Part model, mm, in its own coordinate system. A direction names the side the tool comes from. Round coordinates to 2 decimals unless told otherwise and drop trailing zeros. Loops run counter-clockwise (first coordinate to the right, second up) from the corner with the lowest first, then second, coordinate; pieces in that order, holes last. Notation, with made-up numbers: (-16.5, 81.25) -> (12.5, 81.25) arc R20 cw to (12.5, 105.25) -> close; hole circle Ø11 at (67.25, -39). An arc over 180 degrees is marked (long way). Answer as a JSON object with one key per item and string values. Group by question number.
from build123d import *

# Parameters (mm, degrees)
BOSS_EXTRUDE1_DEPTH = 17
CHAMFER1_SIZE       = 0.5
CUT_EXTRUDE1_DEPTH  = 13
BOSS_EXTRUDE2_START = -2
BOSS_EXTRUDE2_DEPTH = 2
SKETCH2_R           = 1.5499999999999992
SKETCH2_R_2         = 1.550000000000003
SKETCH2_R_3         = 2.5
CUT_EXTRUDE2_DEPTH  = 2
BOSS_EXTRUDE3_DEPTH = 5
FILLET1_R           = 2
FILLET2_R           = 0.5
CHAMFER3_SIZE       = 0.5
CHAMFER3_SIZE2      = 3
CHAMFER4_SIZE       = 1


with BuildPart() as part:
    # Sketch1 → Boss-Extrude1 (new body)
    with BuildSketch(Plane(origin=(0, 0, 0), x_dir=(1, 0, 0), z_dir=(0, 1, 0))):
        with BuildLine():
            ThreePointArc((13.418634843133532, 19.2879126019326), (5.33e-15, 27.035165040773038), (-13.418634843133521, 19.287912601932604))
            Line((-13.418634843133521, 19.2879126019326), (-23.413139720814414, 1.9769223572943453))
            ThreePointArc((-23.413139720814414, 1.976922357294347), (-23.413139720814407, -13.517582520386524), (-9.994504877680875, -21.264834959226956))
            Line((-9.994504877680875, -21.264834959226956), (9.994504877680878, -21.26483495922696))
            ThreePointArc((9.994504877680878, -21.26483495922696), (23.413139720814414, -13.517582520386526), (23.41313972081442, 1.9769223572943506))
            Line((23.41313972081442, 1.9769223572943488), (13.418634843133532, 19.2879126019326))
        make_face()
        with BuildLine():
            Line((-11.469734859267339, 10.663506392859015), (-11.902747561159552, 10.91350639285901))
            Line((-11.902747561159554, 10.91350639285901), (-10.975952641916443, 12.518762281184774))
            Line((-10.975952641916448, 12.518762281184776), (-12.361593287971548, 13.318762281184778))
            Line((-12.361593287971548, 13.318762281184778), (-11.561593287971546, 14.70440292723988))
            Line((-11.561593287971546, 14.70440292723988), (-10.17595264191644, 13.904402927239877))
            Line((-10.175952641916442, 13.904402927239877), (-8.655495122319113, 16.537912601932604))
            ThreePointArc((-8.655495122319113, 16.537912601932604), (1.33e-15, 21.535165040773038), (8.655495122319117, 16.537912601932604))
            Line((8.655495122319117, 16.537912601932604), (10.175952641916444, 13.904402927239877))
            Line((10.175952641916444, 13.904402927239877), (11.561593287971549, 14.70440292723988))
            Line((11.561593287971549, 14.70440292723988), (12.361593287971552, 13.318762281184778))
            Line((12.361593287971552, 13.318762281184778), (10.975952641916452, 12.518762281184776))
            Line((10.975952641916447, 12.518762281184772), (11.902747561159558, 10.91350639285901))
            Line((11.902747561159556, 10.913506392859007), (11.46973485926734, 10.663506392859015))
            Line((11.46973485926734, 10.663506392859015), (14.969734859267339, 4.601328566367944))
            Line((14.969734859267339, 4.601328566367944), (15.402747561159552, 4.851328566367944))
            Line((15.402747561159552, 4.8513285663679415), (18.64999999999999, -0.7730776427056512))
            ThreePointArc((18.64999999999999, -0.7730776427056494), (18.65, -10.767582520386522), (9.994504877680878, -15.764834959226958))
            Line((9.994504877680878, -15.76483495922696), (-9.994504877680871, -15.76483495922696))
            ThreePointArc((-9.994504877680868, -15.76483495922696), (-18.64999999999999, -10.767582520386524), (-18.64999999999999, -0.7730776427056494))
            Line((-18.64999999999999, -0.7730776427056512), (-15.402747561159547, 4.851328566367947))
            Line((-15.40274756115955, 4.851328566367947), (-14.969734859267337, 4.601328566367946))
            Line((-14.969734859267337, 4.601328566367946), (-11.469734859267339, 10.663506392859015))
        make_face(mode=Mode.SUBTRACT)
        with BuildLine():
            Line((13.63479836872844, 11.913506392859018), (14.609798368728441, 10.224756855479358))
            ThreePointArc((14.609798368728436, 10.224756855479354), (16.727137744594316, 9.657417479613473), (16.159798368728428, 7.540078103747593))
            Line((16.15979836872844, 7.5400781037476), (17.13479836872844, 5.851328566367942))
            Line((17.13479836872844, 5.851328566367942), (16.268772964944, 5.351328566367942))
            Line((16.268772964944, 5.351328566367942), (12.768772964944, 11.413506392859018))
            Line((12.768772964944, 11.413506392859018), (13.63479836872844, 11.913506392859018))
        make_face(mode=Mode.SUBTRACT)
        with BuildLine():
            Line((-13.634798368728436, 11.913506392859018), (-12.768772964943997, 11.413506392859018))
            Line((-12.768772964943997, 11.413506392859018), (-16.268772964944, 5.351328566367942))
            Line((-16.268772964944, 5.351328566367942), (-17.13479836872844, 5.851328566367942))
            Line((-17.13479836872844, 5.851328566367942), (-16.159798368728442, 7.540078103747597))
            ThreePointArc((-16.159798368728435, 7.540078103747593), (-16.727137744594312, 9.65741747961347), (-14.60979836872844, 10.224756855479354))
            Line((-14.609798368728441, 10.224756855479356), (-13.634798368728436, 11.913506392859018))
        make_face(mode=Mode.SUBTRACT)
    extrude(amount=BOSS_EXTRUDE1_DEPTH)

    # Chamfer1
    chamfer1_edges = [part.edges().sort_by_distance(p)[0] for p in [
        (-10.175952641916442, 8.5, -13.904402927239877),
        (-10.975952641916447, 8.5, -12.518762281184774),
        (10.97595264191645, 8.5, -12.518762281184774),
        (10.175952641916444, 8.5, -13.904402927239877),
    ]]
    chamfer(chamfer1_edges, length=CHAMFER1_SIZE)

    # Sketch1<3> → Cut-Extrude1 (cut)
    with BuildSketch(Plane(origin=(0, 0, 0), x_dir=(1, 0, 0), z_dir=(0, 1, 0))):
        Polygon((-12.585760263051778, 10.7304936909668), (-13.018772964943997, 10.9804936909668), (-13.518772964943999, 10.114468287182358), (-13.085760263051776, 9.86446828718236), align=None)
        Polygon((-15.08576026305178, 6.400366672044599), (-15.518772964944, 6.650366672044602), (-16.018772964944, 5.784341268260162), (-15.585760263051782, 5.53434126826016), align=None)
        Polygon((13.518772964944, 10.114468287182358), (13.018772964944, 10.9804936909668), (12.585760263051782, 10.7304936909668), (13.08576026305178, 9.86446828718236), align=None)
        Polygon((16.018772964944, 5.784341268260162), (15.518772964944, 6.6503666720445995), (15.085760263051784, 6.400366672044599), (15.585760263051785, 5.53434126826016), align=None)
    extrude(amount=CUT_EXTRUDE1_DEPTH, mode=Mode.SUBTRACT)

    # Sketch1<4> → Boss-Extrude2 (add)
    with BuildSketch(Plane(origin=(0, 0, 0), x_dir=(1, 0, 0), z_dir=(0, 1, 0)).offset(BOSS_EXTRUDE2_START)):
        with BuildLine():
            Line((-13.418634843133521, 19.2879126019326), (-23.413139720814414, 1.976922357294346))
            ThreePointArc((-23.413139720814414, 1.976922357294346), (-23.413139720814407, -13.517582520386522), (-9.994504877680875, -21.264834959226956))
            Line((-9.994504877680875, -21.264834959226956), (9.994504877680878, -21.26483495922696))
            ThreePointArc((9.994504877680878, -21.26483495922696), (23.413139720814414, -13.517582520386522), (23.41313972081442, 1.9769223572943484))
            Line((23.41313972081442, 1.9769223572943484), (13.418634843133532, 19.2879126019326))
            ThreePointArc((13.418634843133532, 19.2879126019326), (3.63e-15, 27.035165040773038), (-13.418634843133521, 19.2879126019326))
        make_face()
    extrude(amount=BOSS_EXTRUDE2_DEPTH)

    # Sketch2 → Cut-Extrude2 (cut)
    # profile 1 of 4: a face of its own
    with BuildSketch(Plane.XZ.offset(2)):
        with Locations(Location((-15.384798368728436, -8.882417479613482, 0), (0, 0, 270))):
            Circle(SKETCH2_R)
    # profile 2 of 4: a face of its own
    with BuildSketch(Plane.XZ.offset(2)):
        with Locations(Location((15.38479836872844, -8.882417479613482, 0), (0, 0, 270))):
            Circle(SKETCH2_R_2)
    # profile 3 of 4: a face of its own
    with BuildSketch(Plane.XZ.offset(2)):
        with Locations(Location((0, 0, 0), (0, 0, 270))):
            Circle(SKETCH2_R_3)
    # profile 4 of 4: a face of its own
    with BuildSketch(Plane.XZ.offset(2)):
        Polygon((5.499999999999999, 21.264834959226956), (5.5, 25.264834959226956), (-5.5, 25.264834959226956), (-5.499999999999999, 21.264834959226956), align=None)
        with BuildLine():
            Line((-1.4999999999999987, 24.264834959226945), (1.4999999999999987, 24.264834959226945))
            ThreePointArc((1.4999999999999987, 24.264834959226945), (2.7499999999999916, 23.014834959226953), (1.4999999999999987, 21.76483495922696))
            Line((1.4999999999999987, 21.76483495922696), (-1.4999999999999987, 21.76483495922696))
            ThreePointArc((-1.4999999999999987, 21.76483495922696), (-2.7499999999999916, 23.014834959226953), (-1.4999999999999987, 24.264834959226945))
        make_face(mode=Mode.SUBTRACT)
    extrude(amount=-CUT_EXTRUDE2_DEPTH, mode=Mode.SUBTRACT)

    # Sketch2<2> → Boss-Extrude3 (add)
    with BuildSketch(Plane.XZ.offset(2)):
        Polygon((-5.499999999999999, 21.264834959226956), (5.499999999999999, 21.264834959226956), (5.5, 25.264834959226956), (-5.5, 25.264834959226956), align=None)
        with BuildLine():
            ThreePointArc((-1.499999999999999, 21.76483495922696), (-2.7499999999999916, 23.014834959226953), (-1.4999999999999987, 24.264834959226945))
            Line((-1.4999999999999987, 24.264834959226945), (1.4999999999999987, 24.264834959226945))
            ThreePointArc((1.499999999999999, 24.264834959226945), (2.7499999999999916, 23.014834959226953), (1.4999999999999987, 21.76483495922696))
            Line((1.4999999999999987, 21.76483495922696), (-1.4999999999999987, 21.76483495922696))
        make_face(mode=Mode.SUBTRACT)
    extrude(amount=-BOSS_EXTRUDE3_DEPTH)

    # Fillet1
    fillet1_edges = [part.edges().sort_by_distance(p)[0] for p in [
        (5.499999999999999, 0.5, 21.264834959226956),
        (-5.499999999999999, 0.5, 21.264834959226956),
    ]]
    fillet(fillet1_edges, radius=FILLET1_R)
    fillet1_2_edges = [part.edges().sort_by_distance(p)[0] for p in [
        (5.5, 0.5, 25.264834959226956),
        (-5.5, 0.5, 25.264834959226956),
    ]]
    fillet(fillet1_2_edges, radius=FILLET1_R - 0.0001)  # a hair under: the kernel refuses the full size

    # Fillet2
    fillet2_edges = [part.edges().sort_by_distance(p)[0] for p in [
        (0, 3, 24.264834959226945),
        (2.7499999999999916, 3, 23.014834959226953),
        (-2.7499999999999916, 3, 23.014834959226953),
        (0, 3, 21.76483495922696),
    ]]
    fillet(fillet2_edges, radius=FILLET2_R - 0.0001)  # a hair under: the kernel refuses the full size

    # Chamfer3
    chamfer3_edges = [part.edges().sort_by_distance(p)[0] for p in [
        (13.21973485926734, 17, -7.63241747961348),
        (-13.219734859267337, 17, -7.63241747961348),
        (14.518772964943999, 17, -8.38241747961348),
        (-14.518772964943999, 17, -8.38241747961348),
    ]]
    chamfer3_side = [part.faces().sort_by_distance(p)[0] for p in [
        (-12.172522474712478, 17, -11.850756469441762),
    ]]
    chamfer(chamfer3_edges, length=CHAMFER3_SIZE, length2=CHAMFER3_SIZE2, reference=chamfer3_side[0])

    # Chamfer4
    chamfer4_edges = [part.edges().sort_by_distance(p)[0] for p in [
        (1.78e-15, 17, 21.26483495922696),
        (23.413139720814414, 17, 13.517582520386522),
        (18.415887281973976, 17, -10.632417479613474),
        (4.44e-15, 17, -27.035165040773038),
        (-18.415887281973966, 17, -10.632417479613473),
        (-23.413139720814407, 17, 13.517582520386526),
        (5.33e-15, -2, -27.035165040773038),
        (23.413139720814414, -2, 13.517582520386526),
        (-8.747252438840437, -2, 21.264834959226956),
        (-23.413139720814407, -2, 13.517582520386524),
        (-18.415887281973966, -2, -10.632417479613473),
        (18.415887281973976, -2, -10.632417479613474),
        (8.747252438840441, -2, 21.26483495922696),
        (0, -2, 25.264834959226956),
        (-4.9142428516949765, -2, 24.67907781092193),
        (4.914242851694976, -2, 24.67907781092193),
        (6.085786437626905, -2, 21.850621396853864),
        (-6.085786437626905, -2, 21.85062139685386),
    ]]
    chamfer(chamfer4_edges, length=CHAMFER4_SIZE - 0.0001)  # a hair under: the kernel refuses the full size


solid = part.part
Item 1: Band-saw the part on A-A, the plane x = 0. Count the separate pieces of the cut face and the enclosed holes in it, plus the area to 3 significant figures.
Item 2: Band-saw the part on C-C, the plane z = -18. List the corners of the cut face in (x, y), plus the area to 3 significant figures.
Item 3: Drop flat-ended pins along their axis: pin 1 Ø3 at (x, z) = (2, 6) entering from +Y; pin 2 Ø5 at (x, y) = (3, 7.5) entering from -Z; pin 3 Ø4 at (y, z) = (7.5, -5.5) entering from -X; pin 4 Ø8 at (x, z) = (5, -15) entering from +Y. Give the stop position or say it passes through.
Item 4: Which spindle directions (+Z, -Z, +X, -X, +Y, -Y) get a long thin tool onto all of the face, cutting with end or side? Do faces 1 (the face through (6.101, 1.028, 21.835)), 2 (the face through (2.75, 0.22, 23.04)), 3 (the face through (14.33, 15.48, -8.22)). Say none if no direction does.
Item 5: Two-plate mould, pull along X, no slides. Class faces 4 (the face through (13.2, 6.9, -7.67)), 5 (the face through (0.215, 16.826, -26.207)), 6 (the face through (-22.8, 16.83, 12.92)): pulls with the +X half, pulls with the -X half, needs draft (parallel to the pull), parting line crosses it, or undercut.
Item 6: Drill centre lines: line 1 (X direction, y = 0.25, z = -6); line 2 (Z direction, x = -17, y = 6.5); line 3 (Z direction, x = -0.5, y = 6.5). Where is each one in solid material? Low to high.
Entries:
{
 "1": {"separate pieces": "3", "enclosed holes": "0", "area": "279 mm²"},
 "2": {"outline": "(-14.16, -1) -> (-13.01, -2) -> (13.01, -2) -> (14.16, -1) -> (14.16, 16) -> (13.01, 17) -> (7.63, 17) -> (7.63, 0) -> (-7.63, 0) -> (-7.63, 17) -> (-13.01, 17) -> (-14.16, 16) -> close", "area": "277 mm²"},
 "3": {"pin 1": "y = 0", "pin 2": "z = -27.03", "pin 3": "x = -22.53", "pin 4": "y = 17"},
 "4": {"face 1": "+Z, +X, +Y, -Y", "face 2": "+Y, -Y", "face 3": "+Y"},
 "5": {"face 4": "undercut", "face 5": "parting line crosses it", "face 6": "pulls with the -X half"},
 "6": {"line 1": "-21.09 to -17.05, -15.32 to -14.16, 14.16 to 15.32, 17.05 to 21.09", "line 2": "-13.08 to -6.08, -5.77 to -2.08, 12.9 to 19.59", "line 3": "-27.03 to -21.52, 15.76 to 21.26"}
}
